Design review of the part built by this model. Coordinates are the model's own, in mm. Give positions to 0.01 mm unless a question says otherwise; leave off trailing zeros. Write each loop counter-clockwise with the first axis right and the second up, starting at its lowest first coordinate (ties: lowest second). Pieces come first, ordered by that corner, then holes.
```python
from build123d import *

# Parameters (mm, degrees)
EXTRUDE1_DEPTH         = 10.414
M8X1_25_TAPPED_HOLE1_D = 6.8


with BuildPart() as part:
    # Sketch1 → Extrude1 (new body)
    with BuildSketch(Plane(origin=(0, 0, 0), x_dir=(1, 0, 0), z_dir=(0, 1, 0))):
        Polygon((3.464101615, 6), (-3.464101615, 6), (-6.92820323, 0), (-3.464101615, -6), (3.464101615, -6), (6.92820323, 0), align=None)
    extrude(amount=EXTRUDE1_DEPTH)

    # M8x1.25 Tapped Hole1 (through all)
    with Locations(Plane(origin=(0, 10.414, 0), x_dir=(-1, 0, 0), z_dir=(0, 1, 0))):
        with Locations((0, 0)):
            Hole(M8X1_25_TAPPED_HOLE1_D / 2)


solid = part.part
```
(1) Consider section A-A, the plane x = 0. Give the boundary of the cut face in (y, z), then the cut area to 3 significant figures.
Resolved:
outline: (0, -6) - (10.41, -6) - (10.41, -3.4) - (0, -3.4) - close; (0, 3.4) - (10.41, 3.4) - (10.41, 6) - (0, 6) - close
area: 54.2 mm2
(2) Consider section B-B, the plane y = 2.25. Give the boundary of the cut face in (x, z), then the cut area to 3 significant figures.
Resolved:
outline: (-6.93, 0) - (-3.46, -6) - (3.46, -6) - (6.93, 0) - (3.46, 6) - (-3.46, 6) - close; hole circle Ø6.8 at (0, 0)
area: 88.4 mm2
(3) Consider section D-D, the plane z = 3.75. Give the boundary of the cut face in (x, y).
Resolved:
outline: (-4.76, 0) - (4.76, 0) - (4.76, 10.41) - (-4.76, 10.41) - close
(4) To check wall thickness, follow L1, parallel to Z at x = 0, y = 4.5; L2, parallel to X at y = 1.25, z = -3; L3, parallel to X at y = 3.5, z = -2. State the ranges of each line that lie inside material, in increasing order.
Resolved:
L1: z = -6 to -3.4, 3.4 to 6
L2: x = -5.2 to -1.6, 1.6 to 5.2
L3: x = -5.77 to -2.75, 2.75 to 5.77
(5) Mouldability with a two-part tool opening along X and no side actions: class faces 1 (the face through (5.172, 5.134, 3.042)), 2 (the face through (-5.22, 5.13, 2.96)), 3 (the face through (3, 10.414, -3)), 4 (the face through (-0.74, 5.13, -3.32)) as pulls with the +X half, pulls with the -X half, needs draft (parallel to the pull), parting line crosses it, or undercut.
Resolved:
face 1: pulls with the +X half
face 2: pulls with the -X half
face 3: needs draft
face 4: undercut
(6) Clearance check with flat-ended pins moving along their axes: P1, Ø6, axis at x = 4, y = 6.5, coming from the -Z side; P2, Ø1, axis at y = 3, z = -1.5, coming from the -X side. State where each tip first meets the part, or that it passes through.
Resolved:
P1: stops at z = -6
P2: stops at x = -6.35
(7) Consider section C-C, the plane z = 1. Give the boundary of the cut face in (x, y), then the cut area to 3 significant figures.
Resolved:
outline: (-6.35, 0) - (-3.25, 0) - (-3.25, 10.41) - (-6.35, 10.41) - close; (3.25, 0) - (6.35, 0) - (6.35, 10.41) - (3.25, 10.41) - close
area: 64.6 mm2
